Could you check a few things on this model? Use its own coordinates, in mm. Coordinates: 2 decimals unless noted, no trailing zeros. Write each loop counter-clockwise with the first axis right and the second up, starting at its lowest first coordinate (ties: lowest second). Pieces come first, ordered by that corner, then holes.
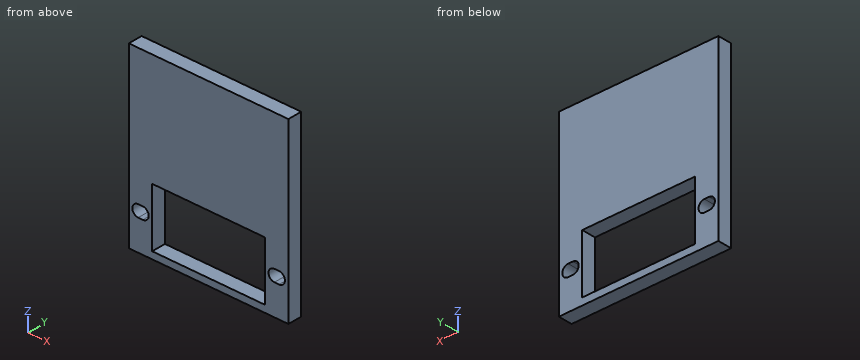
```python
from build123d import *

# Parameters (mm, degrees)
BOSS_EXTRU_1_DEPTH = 3


with BuildPart() as part:
    # Esquisse1 → Boss.-Extru.1 (new body)
    with BuildSketch(Plane(origin=(0, 0, 0), x_dir=(1, 0, 0), z_dir=(0, 1, 0))):
        Polygon((-12.05, 36.5), (0, 36.5), (0, 38), (-17.05, 38), (-17.05, 0), (0, 0), (0, 24), (-12.05, 24), align=None)
        with BuildLine():
            ThreePointArc((-15.05, 29), (-16.3, 30.25), (-15.05, 31.5))
            Line((-15.05, 31.5), (-14.05, 31.5))
            ThreePointArc((-14.05, 31.5), (-12.8, 30.25), (-14.05, 29))
            Line((-14.05, 29), (-15.05, 29))
        make_face(mode=Mode.SUBTRACT)
    boss_extru_1 = extrude(amount=BOSS_EXTRU_1_DEPTH)

    # Symétrie1: Boss.-Extru.1 across plane
    add(boss_extru_1.mirror(Plane(origin=(0, 3, 0), x_dir=(0, 0, 1), z_dir=(-1, 0, 0))))


solid = part.part
```
1. I want a section at A-A on x = 4. Please give me the cut outline in (y, z), plus the area to 3 significant figures.
Verdict:
outline: (0, -38) - (3, -38) - (3, -36.5) - (0, -36.5) - close; (0, -24) - (3, -24) - (3, 0) - (0, 0) - close
area: 76.5 mm2
2. Please list where these lines run through material, in increasing order: line 1 along Z through (x, y) = (-3, 1.55); line 2 along X through (y, z) = (0.5, -28); line 3 along Z through (x, y) = (-13, 0.25).
Verdict:
line 1: z = -38 to -36.5, -24 to 0
line 2: x = -17.05 to -12.05, 12.05 to 17.05
line 3: z = -38 to -30.93, -29.57 to 0
3. I want a section at C-C on y = 0.75. Please give me the cut outline in (x, z), plus the area to 3 significant figures.
Verdict:
outline: (-17.05, -38) - (17.05, -38) - (17.05, 0) - (-17.05, 0) - close; hole (-15.05, -31.5) - (-14.05, -31.5) arc R1.25 ccw to (-14.05, -29) - (-15.05, -29) arc R1.25 ccw to start; hole (-12.05, -36.5) - (12.05, -36.5) - (12.05, -24) - (-12.05, -24) - close; hole (14.05, -31.5) - (15.05, -31.5) arc R1.25 ccw to (15.05, -29) - (14.05, -29) arc R1.25 ccw to start
area: 980 mm2
4. For pin 1 (6 mm diameter, centred on x = 2.5, z = -28.5, fed in from -Y) (3 decimals), with a flat end and sliding along its axis, tell me the tip position at first contact or that it passes through.
Verdict:
pin 1: passes through
5. I want a section at B-B on z = -33.5. Please give me the cut outline in (x, y), plus the area to 3 significant figures.
Verdict:
outline: (-17.05, 0) - (-12.05, 0) - (-12.05, 3) - (-17.05, 3) - close; (12.05, 0) - (17.05, 0) - (17.05, 3) - (12.05, 3) - close
area: 30.0 mm2
